Read the model definition and answer for the solid it produces. Units are mm, in the model's axes. A direction names the side the tool comes from. Round coordinates to 2 decimals unless told otherwise and drop trailing zeros. Loops run counter-clockwise (first coordinate to the right, second up) from the corner with the lowest first, then second, coordinate; pieces in that order, holes last. Notation, with made-up numbers: M 84.5,51 L 102.5,51 A18 cw 102.5,60 Z; hole C 34,71.25 d3. An arc over 180 degrees is marked long. Write each question's results on one line, items separated by ' | '.
```python
from build123d import *

# Parameters (mm, degrees)
RESSALTO_EXTRUS_O1_DEPTH = 13
ESBO_O3_R                = 2.5
CORTE_EXTRUS_O1_DEPTH    = 8
ESBO_O4_R                = 2.5
CORTE_EXTRUS_O2_DEPTH    = 8


with BuildPart() as part:
    # Esboço1 → Ressalto-extrusão1 (new body)
    with BuildSketch(Plane.XY):
        Polygon((3.510692293, 8.611985446), (3.510692293, 6.611985446), (-21.489307707, 6.611985446), (-21.489307707, 31.611985446), (-19.489307707, 31.611985446), (-19.489307707, 8.611985446), align=None)
    extrude(amount=RESSALTO_EXTRUS_O1_DEPTH)

    # Esboço3 → Corte-extrusão1 (cut)
    with BuildSketch(Plane(origin=(-19.489307707, 0, 0), x_dir=(0, 0, -1), z_dir=(1, 0, 0))):
        with Locations(Location((-6.5, 23.611985446, 0), (0, 0, 90))):
            Circle(ESBO_O3_R)
    extrude(amount=-CORTE_EXTRUS_O1_DEPTH, mode=Mode.SUBTRACT)

    # Esboço4 → Corte-extrusão2 (cut)
    with BuildSketch(Plane(origin=(0, 8.611985446, 0), x_dir=(1, 0, 0), z_dir=(0, 1, 0))):
        with Locations(Location((-4.489307707, -6.5, 0), (0, 0, 270))):
            Circle(ESBO_O4_R)
    extrude(amount=-CORTE_EXTRUS_O2_DEPTH, mode=Mode.SUBTRACT)


solid = part.part
```
1. Find section C-C, the plane z = 1.75. Give the vertices of the cut face in (x, y), then the cut area to 3 significant figures.
Completed:
outline: M -21.49,6.61 L 3.51,6.61 L 3.51,8.61 L -19.49,8.61 L -19.49,31.61 L -21.49,31.61 Z | area: 96.0 mm2
2. Determine the mould class of faces 1 (the face through (-9, 6.612, 6)), 2 (the face through (-20.48, 25.92, 5.54)), 3 (the face through (-14, 8, 0)) for opening direction Z: released by +Z, released by -Z, zero draft, split by the parting line, or undercut.
Completed:
face 1: zero draft | face 2: undercut | face 3: released by -Z
3. Find section A-A, the plane z = 6.5. Give the vertices of the cut face in (x, y).
Completed:
outline: M -21.49,6.61 L -6.99,6.61 L -6.99,8.61 L -19.49,8.61 L -19.49,21.11 L -21.49,21.11 Z; M -21.49,26.11 L -19.49,26.11 L -19.49,31.61 L -21.49,31.61 Z; M -1.99,6.61 L 3.51,6.61 L 3.51,8.61 L -1.99,8.61 Z
4. Which of the six approach directions +Z, -Z, +X, -X, +Y, -Y give full straight-line access (tool end or side, diameter ignored) to faces 4 (the face through (-19.489, 20, 6)), 5 (the face through (-5.45, 7.63, 8.81))?
Completed:
face 4: +Z, -Z, +X, +Y | face 5: +Y, -Y
5. Find section B-B, the plane y = 24.5. Give the vertices of the cut face in (x, z).
Completed:
outline: M -21.49,0 L -19.49,0 L -19.49,4.16 L -21.49,4.16 Z; M -21.49,8.84 L -19.49,8.84 L -19.49,13 L -21.49,13 Z
6. Find the intervals of material crossed by L1, parallel to X at y = 7.3, z = 6.5; L2, parallel to X at y = 14.75, z = 1.5; L3, parallel to Y at x = -8.5, z = 1, in increasing order.
Completed:
L1: x = -21.49 to -6.99, -1.99 to 3.51 | L2: x = -21.49 to -19.49 | L3: y = 6.61 to 8.61
7. Find section D-D, the plane y = 16.75. Give the vertices of the cut face in (x, z).
Completed:
outline: M -21.49,0 L -19.49,0 L -19.49,13 L -21.49,13 Z
8. Given P1, Ø4, axis at x = -10, z = 2.5, coming from the +Y side; P2, Ø5, axis at y = 11.5, z = 7, coming from the +X side; P3, Ø4.5, axis at y = 23.61, z = 6.5, coming from the -X side, each flat-ended and moving along its own axis, determine where each tip first touches the part or whether it passes through.
Completed:
P1: stops at y = 8.61 | P2: stops at x = -19.49 | P3: passes through
